For this review, take the finished solid that the model builds, in its own axes (mm). A direction names the side the tool comes from. Give positions to 0.01 mm unless a question says otherwise; leave off trailing zeros. Order: outer loops, then holes, each group sorted by start corner. A loop starts at its lowest first (then second) coordinate and runs counter-clockwise, first axis right, second up. Notation, with made-up numbers: M -17.5,-30 L 23.5,-30 A20 ccw 23.5,-22 Z; hole C 60,55 d4. An arc over 180 degrees is marked long. Use CSV: the item, a comma, the result in double quotes. Start each with the question number.
(1) Wall thickness on L1, parallel to X at y = -85.5, z = 89; L2, parallel to Y at x = 142.5, z = 40.5; L3, parallel to X at y = -183.5, z = 36: over which ranges is each line inside the solid? List them lowest first. Write a range as from..to.
(2) Draft analysis for pull direction X (two halves, no side actions). For faces 1 (the face through (70, -99, 39)), 2 (the face through (-101, 100, 49)), state which applies: pulls with the +X half, pulls with the -X half, needs draft (parallel to the pull), parting line crosses it, or undercut.
(3) Consider section C-C (x = -37). Write out the cut boundary in (y, z), and give its area (3 significant figures).
(4) Consider section A-A (y = -205.5). Write out the cut boundary in (x, z).
(5) Clearance check with flat-ended pins moving along their axes: P1, Ø5.5, axis at x = 130.05, y = -128.93, coming from the -Z side; P2, Ø8.5, axis at x = 64.5, y = -112.5, coming from the +Z side; P3, Ø3, axis at x = 69.95, y = -128.93, coming from the -Z side; P4, Ø3, axis at x = 197, z = 43.5, coming from the +Y side. State where each tip first meets the part, or that it passes through.
(6) Consider section B-B (z = 14.5). Write out the cut boundary in (x, y), and give its area (3 significant figures).
(7) Tool access review of faces 3 (the face through (70, -99, 73)), 4 (the face through (97, -103, 100)), 5 (the face through (135.43, -131.994, 17.39)), 6 (the face through (250, 49, 51)): name each direction out of +Z, -Z, +X, -X, +Y, -Y from which nothing blocks a thin tool from reaching the whole face with its end or side.
```python
from build123d import *

# Parameters (mm, degrees)
SKETCH_1_W               = 200
SKETCH_1_H               = 200
EXTRUDE_1_DEPTH          = 100
CUT_EXTRUDE_1_DEPTH      = 301
CUT_EXTRUDE_1_DEPTH_BACK = 34.3
SKETCH_3_R               = 30
CUT_EXTRUDE_2_DEPTH      = 9
CUT_EXTRUDE_3_REACH      = 302
CUT_EXTRUDE_4_DEPTH      = 55
SKETCH_7_R               = 1.75
CUT_EXTRUDE_7_DEPTH      = 291.373018719
SKETCH_9_W               = 100
SKETCH_9_H               = 200
EXTRUDE_2_DEPTH          = 150
SKETCH_10_W              = 100
SKETCH_10_H              = 200
EXTRUDE_3_DEPTH          = 150
SKETCH_11_W              = 100
SKETCH_11_H              = 100
EXTRUDE_4_DEPTH          = 100
SKETCH_12_W              = 100
SKETCH_12_H              = 100
EXTRUDE_5_DEPTH          = 100


with BuildPart() as part:
    # 草图1 → 凸台-拉伸1 (new body)
    with BuildSketch(Plane.XY):
        with Locations((100, -100)):
            Rectangle(SKETCH_1_W, SKETCH_1_H)
    extrude(amount=EXTRUDE_1_DEPTH)

    # 草图2 → 切除-拉伸1 (cut, two sides: drawn at the far end of the back side and taken through both)
    with BuildSketch(Plane(origin=(0, 0, 0), x_dir=(-1, 0, 0), z_dir=(0, 0, -1)).offset(-CUT_EXTRUDE_1_DEPTH_BACK)):
        with BuildLine():
            Line((-146.25, -84.273215621), (-146.25, -98.874157372))
            Line((-146.25, -98.874157372), (-146.25, -113.475099122))
            ThreePointArc((-146.25, -113.475099122), (-100, -147.374157372), (-53.75, -113.475099122))
            Line((-53.75, -113.475099122), (-53.75, -84.273215621))
            ThreePointArc((-53.75, -84.273215621), (-100, -50.374157372), (-146.25, -84.273215621))
        make_face()
    extrude(amount=CUT_EXTRUDE_1_DEPTH + CUT_EXTRUDE_1_DEPTH_BACK, mode=Mode.SUBTRACT)

    # 草图3 → 切除-拉伸2 (cut)
    with BuildSketch(Plane(origin=(0, 0, 34.3), x_dir=(-1, 0, 0), z_dir=(0, 0, -1))):
        with Locations((-100, -98.874157372)):
            Circle(SKETCH_3_R)
    extrude(amount=-CUT_EXTRUDE_2_DEPTH, mode=Mode.SUBTRACT)

    # 切除-拉伸3: up to this face of the body (flat: up to its plane)
    cut_extrude_3_end = Plane(part.part.faces().sort_by_distance((100, -98.874157372, 43.3))[0])
    # 草图4 → 切除-拉伸3 (cut, up to the picked face)
    with BuildSketch(Plane(origin=(0, 0, 0), x_dir=(-1, 0, 0), z_dir=(0, 0, -1)), mode=Mode.PRIVATE) as cut_extrude_3_sk1:
        with BuildLine():
            Line((-82.891665128, 0), (-117.108334872, 0))
            Line((-117.108334872, 0), (-117.108334872, -53.491838371))
            ThreePointArc((-117.108334872, -53.491838371), (-100, -50.374157372), (-82.891665128, -53.491838371))
            Line((-82.891665128, -53.491838371), (-82.891665128, 0))
        make_face()
    cut_extrude_3_tool1 = split(extrude(cut_extrude_3_sk1.sketch, amount=-CUT_EXTRUDE_3_REACH, mode=Mode.PRIVATE), bisect_by=cut_extrude_3_end, keep=Keep.BOTH, mode=Mode.PRIVATE)
    # 草图4 → 切除-拉伸3 (cut, up to the picked face)
    with BuildSketch(Plane(origin=(0, 0, 0), x_dir=(-1, 0, 0), z_dir=(0, 0, -1)), mode=Mode.PRIVATE) as cut_extrude_3_sk2:
        with BuildLine():
            ThreePointArc((-82.891665128, -53.491838371), (-100, -50.374157372), (-117.108334872, -53.491838371))
            Line((-117.108334872, -53.491838371), (-117.108334872, -74.230600853))
            ThreePointArc((-117.108334872, -74.230600853), (-100, -68.874157372), (-82.891665128, -74.230600853))
            Line((-82.891665128, -74.230600853), (-82.891665128, -53.491838371))
        make_face()
    cut_extrude_3_tool2 = split(extrude(cut_extrude_3_sk2.sketch, amount=-CUT_EXTRUDE_3_REACH, mode=Mode.PRIVATE), bisect_by=cut_extrude_3_end, keep=Keep.BOTH, mode=Mode.PRIVATE)
    # 草图4 → 切除-拉伸3 (cut, up to the picked face)
    with BuildSketch(Plane(origin=(0, 0, 0), x_dir=(-1, 0, 0), z_dir=(0, 0, -1)), mode=Mode.PRIVATE) as cut_extrude_3_sk3:
        with BuildLine():
            ThreePointArc((-82.891665128, -74.230600853), (-100, -68.874157372), (-117.108334872, -74.230600853))
            Line((-117.108334872, -74.230600853), (-117.108334872, -123.517713891))
            ThreePointArc((-117.108334872, -123.517713891), (-100, -128.874157372), (-82.891665128, -123.517713891))
            Line((-82.891665128, -123.517713891), (-82.891665128, -74.230600853))
        make_face()
    cut_extrude_3_tool3 = split(extrude(cut_extrude_3_sk3.sketch, amount=-CUT_EXTRUDE_3_REACH, mode=Mode.PRIVATE), bisect_by=cut_extrude_3_end, keep=Keep.BOTH, mode=Mode.PRIVATE)
    # 草图4 → 切除-拉伸3 (cut, up to the picked face)
    with BuildSketch(Plane(origin=(0, 0, 0), x_dir=(-1, 0, 0), z_dir=(0, 0, -1)), mode=Mode.PRIVATE) as cut_extrude_3_sk4:
        with BuildLine():
            ThreePointArc((-82.891665128, -123.517713891), (-100, -128.874157372), (-117.108334872, -123.517713891))
            Line((-117.108334872, -123.517713891), (-117.108334872, -144.256476373))
            ThreePointArc((-117.108334872, -144.256476373), (-100, -147.374157372), (-82.891665128, -144.256476373))
            Line((-82.891665128, -144.256476373), (-82.891665128, -123.517713891))
        make_face()
    cut_extrude_3_tool4 = split(extrude(cut_extrude_3_sk4.sketch, amount=-CUT_EXTRUDE_3_REACH, mode=Mode.PRIVATE), bisect_by=cut_extrude_3_end, keep=Keep.BOTH, mode=Mode.PRIVATE)
    # 草图4 → 切除-拉伸3 (cut, up to the picked face)
    with BuildSketch(Plane(origin=(0, 0, 0), x_dir=(-1, 0, 0), z_dir=(0, 0, -1)), mode=Mode.PRIVATE) as cut_extrude_3_sk5:
        with BuildLine():
            ThreePointArc((-82.891665128, -144.256476373), (-100, -147.374157372), (-117.108334872, -144.256476373))
            Line((-117.108334872, -144.256476373), (-117.108334872, -200))
            Line((-117.108334872, -200), (-82.891665128, -200))
            Line((-82.891665128, -200), (-82.891665128, -144.256476373))
        make_face()
    cut_extrude_3_tool5 = split(extrude(cut_extrude_3_sk5.sketch, amount=-CUT_EXTRUDE_3_REACH, mode=Mode.PRIVATE), bisect_by=cut_extrude_3_end, keep=Keep.BOTH, mode=Mode.PRIVATE)
    add(cut_extrude_3_tool1.solids().sort_by(Axis((100, -25.708145, 0), (0, 0, 1)))[0], mode=Mode.SUBTRACT)
    add(cut_extrude_3_tool2.solids().sort_by(Axis((100, -61.037282, 0), (0, 0, 1)))[0], mode=Mode.SUBTRACT)
    add(cut_extrude_3_tool3.solids().sort_by(Axis((100, -98.874157, 0), (0, 0, 1)))[0], mode=Mode.SUBTRACT)
    add(cut_extrude_3_tool4.solids().sort_by(Axis((100, -136.711033, 0), (0, 0, 1)))[0], mode=Mode.SUBTRACT)
    add(cut_extrude_3_tool5.solids().sort_by(Axis((100, -173.166361, 0), (0, 0, 1)))[0], mode=Mode.SUBTRACT)

    # 草图6 → 切除-拉伸4 (cut)
    with BuildSketch(Plane.XY.offset(100)):
        with BuildLine():
            Line((82.891665128, -74.230600853), (82.891665128, -53.491838371))
            ThreePointArc((82.891665128, -53.491838371), (64.780077431, -65.530386526), (53.75, -84.273215621))
            Line((53.75, -84.273215621), (53.75, -113.475099122))
            ThreePointArc((53.75, -113.475099122), (64.780077431, -132.217928217), (82.891665128, -144.256476373))
            Line((82.891665128, -144.256476373), (82.891665128, -123.517713891))
            ThreePointArc((82.891665128, -123.517713891), (70, -98.874157372), (82.891665128, -74.230600853))
        make_face()
        with BuildLine():
            Line((117.108334872, -53.491838371), (117.108334872, -74.230600853))
            ThreePointArc((117.108334872, -74.230600853), (130, -98.874157372), (117.108334872, -123.517713891))
            Line((117.108334872, -123.517713891), (117.108334872, -144.256476373))
            ThreePointArc((117.108334872, -144.256476373), (135.219922569, -132.217928217), (146.25, -113.475099122))
            Line((146.25, -113.475099122), (146.25, -84.273215621))
            ThreePointArc((146.25, -84.273215621), (135.219922569, -65.530386526), (117.108334872, -53.491838371))
        make_face()
    extrude(amount=-CUT_EXTRUDE_4_DEPTH, mode=Mode.SUBTRACT)

    # 草图7 → 切除-拉伸7 (cut, through all)
    with BuildSketch(Plane(origin=(0, 0, 34.3), x_dir=(-1, 0, 0), z_dir=(0, 0, -1))):
        with Locations((-142.5, -98.874157372)):
            Circle(SKETCH_7_R)
        with Locations((-130.0520382, -68.822119171)):
            Circle(SKETCH_7_R)
        with Locations((-69.9479618, -68.822119171)):
            Circle(SKETCH_7_R)
        with Locations((-57.5, -98.874157372)):
            Circle(SKETCH_7_R)
        with Locations((-69.9479618, -128.926195572)):
            Circle(SKETCH_7_R)
        with Locations((-130.0520382, -128.926195572)):
            Circle(SKETCH_7_R)
    extrude(amount=-CUT_EXTRUDE_7_DEPTH, mode=Mode.SUBTRACT)

    # 草图9 → 凸台-拉伸2 (add)
    with BuildSketch(Plane.ZY):
        with Locations((50, -100)):
            Rectangle(SKETCH_9_W, SKETCH_9_H)
    extrude(amount=EXTRUDE_2_DEPTH)

    # 草图10 → 凸台-拉伸3 (add)
    with BuildSketch(Plane(origin=(200, 0, 0), x_dir=(0, 0, -1), z_dir=(1, 0, 0))):
        with Locations((-50, -100)):
            Rectangle(SKETCH_10_W, SKETCH_10_H)
    extrude(amount=EXTRUDE_3_DEPTH)

    # 草图11 → 凸台-拉伸4 (add)
    with BuildSketch(Plane.XZ.offset(200)):
        with Locations((-100, 50)):
            Rectangle(SKETCH_11_W, SKETCH_11_H)
        with Locations((300, 50)):
            Rectangle(SKETCH_11_W, SKETCH_11_H)
    extrude(amount=EXTRUDE_4_DEPTH)

    # 草图12 → 凸台-拉伸5 (add)
    with BuildSketch(Plane(origin=(0, 0, 0), x_dir=(1, 0, 0), z_dir=(0, 1, 0))):
        with Locations((300, -50)):
            Rectangle(SKETCH_12_W, SKETCH_12_H)
        with Locations((-100, -50)):
            Rectangle(SKETCH_12_W, SKETCH_12_H)
    extrude(amount=EXTRUDE_5_DEPTH)


solid = part.part
```
Check result:
1,L1,"x = -150..53.75, 73.15..126.85, 146.25..350"
1,L2,"y = -200..-100.62, -97.12..0"
1,L3,"x = -150..82.89, 117.11..350"
2,face 1,"undercut"
2,face 2,"needs draft"
3,outline,"M -200,0 L 0,0 L 0,100 L -200,100 Z"
3,area,"20,000 mm^2"
4,outline,"M -150,0 L -50,0 L -50,100 L -150,100 Z; M 250,0 L 350,0 L 350,100 L 250,100 Z"
5,P1,"stops at z = 34.3"
5,P2,"stops at z = 45"
5,P3,"passes through"
5,P4,"stops at y = 0"
6,outline,"M -150,-300 L -50,-300 L -50,-200 L 82.89,-200 L 82.89,-144.26 A48.5 cw 53.75,-113.48 L 53.75,-84.27 A48.5 cw 82.89,-53.49 L 82.89,0 L -50,0 L -50,100 L -150,100 Z; M 117.11,-200 L 250,-200 L 250,-300 L 350,-300 L 350,100 L 250,100 L 250,0 L 117.11,0 L 117.11,-53.49 A48.5 cw 146.25,-84.27 L 146.25,-113.48 A48.5 cw 117.11,-144.26 Z"
6,area,"129,000 mm^2"
7,face 3,"+Z"
7,face 4,"+Z, +X, -X, +Y, -Y"
7,face 5,"-Z"
7,face 6,"+Z, -Z, +Y"
